```python
from build123d import *

# Parameters (mm, degrees)
F1_DEPTH = 25.4


# Not quite as in the source:
# - a feature of the source that left no trace in its solid (it failed there, or was rolled back) is left out


with BuildPart() as f1:
    # F0 (on Front) → F1 (new body)
    with BuildSketch(Plane.XZ):
        with BuildLine():
            ThreePointArc((-79.7143682919, -10.9044297796), (-77.1623604825, -5.7155262496), (-76.2847367633, 0))
            ThreePointArc((-76.2847367633, 0), (-77.1623604825, 5.7155262496), (-79.7143682919, 10.9044297796))
            ThreePointArc((-79.7143682919, 10.9044297796), (-114.3847367633, 0), (-79.7143682919, -10.9044297796))
        make_face()
        Polygon((-82.6373805848, -0.2591255978), (-86.5395795737, -9.1616161244), (-95.5938623611, -12.6973561785), (-104.4963528877, -8.7951571896), (-108.0320929418, 0.2591255978), (-104.1298939529, 9.1616161244), (-95.0756111655, 12.6973561785), (-86.1731206389, 8.7951571896), align=None, mode=Mode.SUBTRACT)
        with BuildLine():
            ThreePointArc((-79.7143682919, 10.9044297796), (-77.1623604825, 5.7155262496), (-76.2847367633, 0))
            ThreePointArc((-76.2847367633, 0), (-77.1623604825, -5.7155262496), (-79.7143682919, -10.9044297796))
            Line((-79.7143682919, -10.9044297796), (78.8772994949, -10.9044297796))
            ThreePointArc((78.8772994949, -10.9044297796), (76.4175133383, 0), (78.8772994949, 10.9044297796))
            Line((78.8772994949, 10.9044297796), (-79.7143682919, 10.9044297796))
        make_face()
        with BuildLine():
            ThreePointArc((-59.6665927425, -6.3275160443), (-65.9941087868, 0), (-59.6665927425, 6.3275160443))
            Line((-59.6665927425, 6.3275160443), (59.6665927425, 6.3275160443))
            ThreePointArc((59.6665927425, 6.3275160443), (65.9941087868, 0), (59.6665927425, -6.3275160443))
            Line((59.6665927425, -6.3275160443), (-59.6665927425, -6.3275160443))
        make_face(mode=Mode.SUBTRACT)
        with BuildLine():
            ThreePointArc((119.1980874489, 18.5223012497), (97.1020716916, 24.9584576863), (78.8772994949, 10.9044297796))
            ThreePointArc((78.8772994949, 10.9044297796), (76.4175133383, 0), (78.8772994949, -10.9044297796))
            ThreePointArc((78.8772994949, -10.9044297796), (104.5265574803, -25.2551198737), (126.5485838124, -5.7908680873))
            Line((126.5485838124, -5.7908680873), (117.6493461886, -8.4813364867))
            Line((117.6493461886, -8.4813364867), (103.0614445864, -12.8916343049))
            ThreePointArc((103.0614445864, -12.8916343049), (95.3234776063, -12.1222036637), (90.3959783062, -6.1065651155))
            Line((90.3959783062, -6.1065651155), (88.9258790335, -1.2439312481))
            ThreePointArc((88.9258790335, -1.2439312481), (89.6953096746, 6.494035732), (95.7109482229, 11.4215350322))
            Line((95.7109482229, 11.4215350322), (110.2988498251, 15.8318328503))
            Line((110.2988498251, 15.8318328503), (119.1980874489, 18.5223012497))
        make_face()
    extrude(amount=F1_DEPTH)


solid = f1.part
```
Design review of the part built by this model. Coordinates are the model's own, in mm. A direction names the side the tool comes from. Give positions to 0.01 mm unless a question says otherwise; leave off trailing zeros. Order: outer loops, then holes, each group sorted by start corner. A loop starts at its lowest first (then second) coordinate and runs counter-clockwise, first axis right, second up. Notation, with made-up numbers: (33.5, -13.75) -> (80.5, -13.75) arc R15 ccw to (80.5, 3.25) -> close; hole circle Ø6 at (-12, 18.25). An arc over 180 degrees is marked (long way). Write each question's results on one line, items separated by ' | '. Start each with the question number.
Q1. Add section C-C on z = -15.5. Give the boundary of the cut face in (x, y), and give its area (3 significant figures).
Q2. Add section B-B on x = 5.5. Give the boundary of the cut face in (y, z), and give its area (3 significant figures).
Q3. Add section A-A on y = -12. Give the boundary of the cut face in (x, z).
Q4. Machinability: for faces 1 (the flat face through (-2, -13, -10.904)), 2 (the flat face through (-84.43, -12.52, 4.33)), 3 (the cylindrical face through (89.643, -12.522, 6.395)), 4 (the flat face through (14, -25.4, -7)), 5 (the flat face through (1, -13, 10.904)), which of the approach directions +Z, -Z, +X, -X, +Y, -Y give a long, thin tool a straight path to every point of the face, cutting with its end or side? Answer none if there is none.
Q5. For pin 1 (2 mm diameter, centred on x = 64, y = -13.5, fed in from +Z); pin 2 (3 mm diameter, centred on y = -21, z = 19, fed in from +X); pin 3 (5 mm diameter, centred on x = -74, y = -4, fed in from -Z); pin 4 (8 mm diameter, centred on x = -69.5, z = 4.5, fed in from +Y), all flat-tipped, find the tip position at first contact; note any pin that passes through.
Q6. Wall thickness on L1, parallel to Z at x = 51, y = -12.5; L2, parallel to X at y = -17.75, z = -5; L3, parallel to X at y = -12.25, z = 3.5: over which ranges is each line inside the solid? List them lowest first. Write a range as from..to.
Found:
1) outline: (-106.41, -25.4) -> (-84.26, -25.4) -> (-84.26, 0) -> (-106.41, 0) -> close; (81.7, -25.4) -> (121.94, -25.4) -> (121.94, 0) -> (81.7, 0) -> close | area: 1,580 mm2
2) outline: (-25.4, -10.9) -> (0, -10.9) -> (0, -6.33) -> (-25.4, -6.33) -> close; (-25.4, 6.33) -> (0, 6.33) -> (0, 10.9) -> (-25.4, 10.9) -> close | area: 233 mm2
3) outline: (-79.71, -10.9) -> (78.88, -10.9) arc R25.4 ccw to (126.55, -5.79) -> (103.06, -12.89) arc R10.16 cw to (90.4, -6.11) -> (88.93, -1.24) arc R10.16 cw to (95.71, 11.42) -> (119.2, 18.52) arc R25.4 ccw to (78.88, 10.9) -> (-79.71, 10.9) arc R19.05 ccw (long way) to start; hole (-108.03, 0.26) -> (-104.5, -8.8) -> (-95.59, -12.7) -> (-86.54, -9.16) -> (-82.64, -0.26) -> (-86.17, 8.8) -> (-95.08, 12.7) -> (-104.13, 9.16) -> close; hole (-59.67, -6.33) -> (59.67, -6.33) arc R6.33 ccw to (59.67, 6.33) -> (-59.67, 6.33) arc R6.33 ccw to start
4) face 1: -Z, +Y, -Y | face 2: +Y, -Y | face 3: +X, +Y, -Y | face 4: +Z, -Z, +X, -X, -Y | face 5: +Z, +Y, -Y
5) pin 1: stops at z = 10.9 | pin 2: stops at x = 119.2 | pin 3: stops at z = -10.9 | pin 4: stops at y = 0
6) L1: z = -10.9..-6.33, 6.33..10.9 | L2: x = -113.72..-105.98, -84.72..-63.54, 63.54..90.06 | L3: x = -114.06..-106.61, -84.11..-64.94, 64.94..88.65
